Build history of the part. All positions in model axes, mm. A direction names the side the tool comes from. Round coordinates to 2 decimals unless told otherwise and drop trailing zeros. Write each loop counter-clockwise with the first axis right and the second up, starting at its lowest first coordinate (ties: lowest second). Pieces come first, ordered by that corner, then holes. Notation, with made-up numbers: (74.25, 11.5) -> (100.25, 11.5) arc R19 cw to (100.25, 46.5) -> close; hole circle Ø11 at (71, 61.25). An arc over 180 degrees is marked (long way). Answer as CSV lines item,"result".
from build123d import *

# Parameters (mm, degrees)
SKETCH1_R                    = 14
BOSS_EXTRUDE1_DEPTH          = 36
SKETCH1_3_R                  = 2
BOSS_EXTRUDE2_DEPTH          = 15
BOSS_EXTRUDE3_START          = -38
SKETCH1_4_R                  = 2
BOSS_EXTRUDE3_DEPTH          = 2
CHAMFER1_SIZE                = 0.5
CHAMFER2_SIZE                = 2
FILLET1_SIZE                 = 2
FILLET1_SIZE_2               = 4
M3X0_5_TAPPED_HOLE2_D        = 2.5
M3X0_5_TAPPED_HOLE2_DEPTH    = 4
M3X0_5_TAPPED_HOLE2_TIP      = 0.751075774
M3X0_5_TAPPED_HOLE3_D        = 2.5
M3X0_5_TAPPED_HOLE3_DEPTH    = 4
M3X0_5_TAPPED_HOLE3_TIP      = 0.751075774
M2_5X0_45_TAPPED_HOLE1_D     = 2.05
M2_5X0_45_TAPPED_HOLE1_DEPTH = 4
M2_5X0_45_TAPPED_HOLE1_TIP   = 0.615882135


with BuildPart() as part:
    # Sketch1 → Boss-Extrude1 (new body)
    with BuildSketch(Plane(origin=(0, 0, 0), x_dir=(1, 0, 0), z_dir=(0, 1, 0))):
        with Locations(Location((0, 0, 0), (0, 0, 270))):
            Circle(SKETCH1_R)
    extrude(amount=-BOSS_EXTRUDE1_DEPTH)

    # Sketch1<3> → Boss-Extrude2 (add)
    with BuildSketch(Plane(origin=(0, 0, 0), x_dir=(1, 0, 0), z_dir=(0, 1, 0))):
        with Locations(Location((0, 0, 0), (0, 0, 270))):
            Circle(SKETCH1_3_R)
    extrude(amount=BOSS_EXTRUDE2_DEPTH)

    # Sketch1<4> → Boss-Extrude3 (add)
    with BuildSketch(Plane(origin=(0, 0, 0), x_dir=(1, 0, 0), z_dir=(0, 1, 0)).offset(BOSS_EXTRUDE3_START)):
        with Locations(Location((0, 0, 0), (0, 0, 270))):
            Circle(SKETCH1_4_R)
    extrude(amount=BOSS_EXTRUDE3_DEPTH)

    # Chamfer1
    chamfer1_edges = [part.edges().sort_by_distance(p)[0] for p in [
        (0, -38, -2),
        (0, 15, -2),
    ]]
    chamfer(chamfer1_edges, length=CHAMFER1_SIZE)

    # Chamfer2
    chamfer2_edges = [part.edges().sort_by_distance(p)[0] for p in [
        (0, 0, -14),
    ]]
    chamfer(chamfer2_edges, length=CHAMFER2_SIZE)

    # Fillet1
    # an asymmetric fillet: 4, 2 mm, written as the material it takes off along each edge
    with BuildSketch(Plane(origin=(0, -36, 0), x_dir=(0, 0, 1), z_dir=(-1, 0, 0))) as fillet1_piece_1:
        with BuildLine():
            Bezier((14, FILLET1_SIZE), (14, 0), (14 - FILLET1_SIZE_2, 0), weights=[1, 0.707106781, 1])
            Line((14 - FILLET1_SIZE_2, 0), (14, 0))
            Line((14, 0), (14, FILLET1_SIZE))
        make_face()
    revolve(axis=Axis((0, -36, 0), (0, 1, 0)), mode=Mode.SUBTRACT)

    # M3x0.5 Tapped Hole2
    with Locations(Plane(origin=(0, 0, 0), x_dir=(1, 0, 0), z_dir=(0, 1, 0))):
        with Locations((9.5, 0), (0, 8), (0, -8), (-9.5, 0)):
            Hole(M3X0_5_TAPPED_HOLE2_D / 2, depth=M3X0_5_TAPPED_HOLE2_DEPTH)
            with Locations((0, 0, -(M3X0_5_TAPPED_HOLE2_DEPTH + M3X0_5_TAPPED_HOLE2_TIP / 2))):  # 118° drill point
                Cone(0, M3X0_5_TAPPED_HOLE2_D / 2, M3X0_5_TAPPED_HOLE2_TIP, mode=Mode.SUBTRACT)

    # M3x0.5 Tapped Hole3
    with Locations(Plane.XZ.offset(36)):
        with Locations((6, 0), (-6, 0)):
            Hole(M3X0_5_TAPPED_HOLE3_D / 2, depth=M3X0_5_TAPPED_HOLE3_DEPTH)
            with Locations((0, 0, -(M3X0_5_TAPPED_HOLE3_DEPTH + M3X0_5_TAPPED_HOLE3_TIP / 2))):  # 118° drill point
                Cone(0, M3X0_5_TAPPED_HOLE3_D / 2, M3X0_5_TAPPED_HOLE3_TIP, mode=Mode.SUBTRACT)

    # M2.5x0.45 Tapped Hole1
    with Locations(Plane(origin=(0, -36, 0), x_dir=(-1, 0, 0), z_dir=(0, -1, 0))):
        with Locations((0, 6), (5.196152423, -3), (-5.196152423, -3)):
            Hole(M2_5X0_45_TAPPED_HOLE1_D / 2, depth=M2_5X0_45_TAPPED_HOLE1_DEPTH)
            with Locations((0, 0, -(M2_5X0_45_TAPPED_HOLE1_DEPTH + M2_5X0_45_TAPPED_HOLE1_TIP / 2))):  # 118° drill point
                Cone(0, M2_5X0_45_TAPPED_HOLE1_D / 2, M2_5X0_45_TAPPED_HOLE1_TIP, mode=Mode.SUBTRACT)


solid = part.part
1. Drop flat-ended pins along their axis: pin 1 Ø2 at (x, z) = (10, -5.5) entering from -Y; pin 2 Ø12 at (y, z) = (-10.5, 7.5) entering from -X; pin 3 Ø1 at (x, y) = (-7, -32) entering from -Z. Give the stop position or say it passes through.
Results found:
pin 1,"stops at y = -35.99"
pin 2,"stops at x = -13.92"
pin 3,"stops at z = -12.4"
2. Cut at A-A, the plane y = -27. Write the cut outline in (x, z).
Results found:
outline,"circle Ø28 at (0, 0)"
3. Probe line 1 along X through (y, z) = (-34.05, 0); line 2 along Z through (x, y) = (-6, -32.8); line 3 along Z through (x, y) = (0, -1). List the from-to ranges inside material, lowest first.
Results found:
line 1,"x = -14 to -7.25, -4.75 to 4.75, 7.25 to 14"
line 2,"z = -12.65 to -1.25, 1.25 to 2.36, 3.64 to 12.65"
line 3,"z = -13 to -9.25, -6.75 to 6.75, 9.25 to 13"
4. Mould opens along X. For faces 1 (the flat face through (2.4, -36, -0.1)), 2 (the cylindrical face through (-6.22, -33.97, 2.95)), 3 (the conical face through (-6.22, -31.38, 0.01)), 4 (the cylindrical face through (-2, -37, 0)) say: +X half, -X half, draft (parallel to the pull), parting line (faces both ways), or undercut.
Results found:
face 1,"draft"
face 2,"undercut"
face 3,"undercut"
face 4,"parting line"
5. Which spindle directions (+Z, -Z, +X, -X, +Y, -Y) get a long thin tool onto all of the face, cutting with end or side? Do faces 5 (the cylindrical face through (-4.75, -33.97, 0.05)), 6 (the cylindrical face through (0.27, -2.03, 9.22)). Say none if no direction does.
Results found:
face 5,"-Y"
face 6,"+Y"
